Autodesk Inventor part; units mm, degrees
ref_plane "YZ Plane" through (0, 0, 0) normal (1, 0, 0) x (0, 1, 0)
ref_plane "XZ Plane" through (0, 0, 0) normal (0, 1, 0) x (-1, 0, 0)
ref_plane "XY Plane" through (0, 0, 0) normal (0, 0, 1) x (1, 0, 0)
sketch "Sketch1" plane through (0, 0, 0) normal (0, 1, 0) x (-1, 0, 0)
  arc A0 (-5.66, 120.49) -> (-5.66, 124.19) centre (-5.66, 122.34) ccw
  arc A1 (-5.66, 124.19) -> (-5.66, 120.49) centre (-5.66, 122.34) ccw
  arc A2 (5.66, 120.49) -> (5.66, 124.19) centre (5.66, 122.34) ccw
  arc A3 (5.66, 124.19) -> (5.66, 120.49) centre (5.66, 122.34) ccw
  arc A4 (0, 134.15) -> (0, 137.85) centre (0, 136) ccw
  arc A5 (0, 137.85) -> (0, 134.15) centre (0, 136) ccw
  arc A6 (-5.66, 131.81) -> (-5.66, 135.51) centre (-5.66, 133.66) ccw
  arc A7 (-5.66, 135.51) -> (-5.66, 131.81) centre (-5.66, 133.66) ccw
  arc A8 (5.66, 131.81) -> (5.66, 135.51) centre (5.66, 133.66) ccw
  arc A9 (5.66, 135.51) -> (5.66, 131.81) centre (5.66, 133.66) ccw
  arc A10 (8, 126.15) -> (8, 129.85) centre (8, 128) ccw
  arc A11 (8, 129.85) -> (8, 126.15) centre (8, 128) ccw
  arc A12 (0, 124) -> (0, 132) centre (0, 128) ccw
  arc A13 (0, 132) -> (0, 124) centre (0, 128) ccw
  arc A14 (-8, 126.15) -> (-8, 129.85) centre (-8, 128) ccw
  arc A15 (-8, 129.85) -> (-8, 126.15) centre (-8, 128) ccw
  arc A16 (0, 118.15) -> (0, 121.85) centre (0, 120) ccw
  arc A17 (0, 121.85) -> (0, 118.15) centre (0, 120) ccw
  arc A18 (-5.66, 195.81) -> (-5.66, 199.51) centre (-5.66, 197.66) ccw
  arc A19 (-5.66, 199.51) -> (-5.66, 195.81) centre (-5.66, 197.66) ccw
  arc A20 (-5.66, 184.49) -> (-5.66, 188.19) centre (-5.66, 186.34) ccw
  arc A21 (-5.66, 188.19) -> (-5.66, 184.49) centre (-5.66, 186.34) ccw
  arc A22 (5.66, 184.49) -> (5.66, 188.19) centre (5.66, 186.34) ccw
  arc A23 (5.66, 188.19) -> (5.66, 184.49) centre (5.66, 186.34) ccw
  arc A24 (5.66, 195.81) -> (5.66, 199.51) centre (5.66, 197.66) ccw
  arc A25 (5.66, 199.51) -> (5.66, 195.81) centre (5.66, 197.66) ccw
  arc A26 (8, 190.15) -> (8, 193.85) centre (8, 192) ccw
  arc A27 (8, 193.85) -> (8, 190.15) centre (8, 192) ccw
  arc A28 (-8, 190.15) -> (-8, 193.85) centre (-8, 192) ccw
  arc A29 (-8, 193.85) -> (-8, 190.15) centre (-8, 192) ccw
  arc A30 (0, 198.15) -> (0, 201.85) centre (0, 200) ccw
  arc A31 (0, 201.85) -> (0, 198.15) centre (0, 200) ccw
  arc A32 (0, 182.15) -> (0, 185.85) centre (0, 184) ccw
  arc A33 (0, 185.85) -> (0, 182.15) centre (0, 184) ccw
  arc A34 (0, 188) -> (0, 196) centre (0, 192) ccw
  arc A35 (0, 196) -> (0, 188) centre (0, 192) ccw
  arc A36 (8, 158.15) -> (8, 161.85) centre (8, 160) ccw
  arc A37 (8, 161.85) -> (8, 158.15) centre (8, 160) ccw
  arc A38 (-8, 158.15) -> (-8, 161.85) centre (-8, 160) ccw
  arc A39 (-8, 161.85) -> (-8, 158.15) centre (-8, 160) ccw
  arc A40 (0, 166.15) -> (0, 169.85) centre (0, 168) ccw
  arc A41 (0, 169.85) -> (0, 166.15) centre (0, 168) ccw
  arc A42 (0, 150.15) -> (0, 153.85) centre (0, 152) ccw
  arc A43 (0, 153.85) -> (0, 150.15) centre (0, 152) ccw
  arc A44 (0, 156) -> (0, 164) centre (0, 160) ccw
  arc A45 (0, 164) -> (0, 156) centre (0, 160) ccw
  arc A46 (-5.66, 248.49) -> (-5.66, 252.19) centre (-5.66, 250.34) ccw
  arc A47 (-5.66, 252.19) -> (-5.66, 248.49) centre (-5.66, 250.34) ccw
  arc A48 (5.66, 248.49) -> (5.66, 252.19) centre (5.66, 250.34) ccw
  arc A49 (5.66, 252.19) -> (5.66, 248.49) centre (5.66, 250.34) ccw
  arc A50 (0, 262.15) -> (0, 265.85) centre (0, 264) ccw
  arc A51 (0, 265.85) -> (0, 262.15) centre (0, 264) ccw
  arc A52 (-5.66, 259.81) -> (-5.66, 263.51) centre (-5.66, 261.66) ccw
  arc A53 (-5.66, 263.51) -> (-5.66, 259.81) centre (-5.66, 261.66) ccw
  arc A54 (5.66, 259.81) -> (5.66, 263.51) centre (5.66, 261.66) ccw
  arc A55 (5.66, 263.51) -> (5.66, 259.81) centre (5.66, 261.66) ccw
  arc A56 (8, 254.15) -> (8, 257.85) centre (8, 256) ccw
  arc A57 (8, 257.85) -> (8, 254.15) centre (8, 256) ccw
  arc A58 (0, 252) -> (0, 260) centre (0, 256) ccw
  arc A59 (0, 260) -> (0, 252) centre (0, 256) ccw
  arc A60 (8, 222.15) -> (8, 225.85) centre (8, 224) ccw
  arc A61 (8, 225.85) -> (8, 222.15) centre (8, 224) ccw
  arc A62 (-8, 222.15) -> (-8, 225.85) centre (-8, 224) ccw
  arc A63 (-8, 225.85) -> (-8, 222.15) centre (-8, 224) ccw
  arc A64 (0, 230.15) -> (0, 233.85) centre (0, 232) ccw
  arc A65 (0, 233.85) -> (0, 230.15) centre (0, 232) ccw
  arc A66 (0, 214.15) -> (0, 217.85) centre (0, 216) ccw
  arc A67 (0, 217.85) -> (0, 214.15) centre (0, 216) ccw
  arc A68 (0, 220) -> (0, 228) centre (0, 224) ccw
  arc A69 (0, 228) -> (0, 220) centre (0, 224) ccw
  arc A70 (0, 140) -> (0, 148) centre (0, 144) ccw
  arc A71 (0, 148) -> (0, 140) centre (0, 144) ccw
  arc A72 (0.1754, 172) -> (0.1754, 180) centre (0.1754, 176) ccw
  arc A73 (0.1754, 180) -> (0.1754, 172) centre (0.1754, 176) ccw
  arc A74 (0, 204) -> (0, 212) centre (0, 208) ccw
  arc A75 (0, 212) -> (0, 204) centre (0, 208) ccw
  arc A76 (0, 236) -> (0, 244) centre (0, 240) ccw
  arc A77 (0, 244) -> (0, 236) centre (0, 240) ccw
  arc A78 (-8, 254.15) -> (-8, 257.85) centre (-8, 256) ccw
  arc A79 (-8, 257.85) -> (-8, 254.15) centre (-8, 256) ccw
  arc A80 (0, 246.15) -> (0, 249.85) centre (0, 248) ccw
  arc A81 (0, 249.85) -> (0, 246.15) centre (0, 248) ccw
  arc A82 (13.5, 256) -> (0, 269.5) centre (0, 256) ccw
  arc A83 (0, 269.5) -> (-13.5, 256) centre (0, 256) ccw
  line L0 (-13.5, 256) -> (-13.5, 128)
  line L1 (13.5, 128) -> (13.5, 256)
  arc A84 (2.852, 141.1953) -> (-2.852, 141.1953) centre (0, 128) ccw
  arc A85 (-13.5, 128) -> (13.5, 128) centre (0, 128) ccw
  point P0 (0, 0)
  point P1 (0, 128)
extrude "Extrusion1" add sketch "Sketch1" along normal blind 2
sketch "Sketch2" plane through (0, 2, 0) normal (0, 1, 0) x (1, 0, 0)
  line L0 (-13.5, -128) -> (-13.5, -256)
  line L1 (-13.5, -148.6948) -> (13.5, -148.6948)
  line L2 (13.5, -148.6948) -> (13.5, -110.804)
  line L3 (13.5, -110.804) -> (-13.5, -110.804)
  line L4 (-13.5, -110.804) -> (-13.5, -148.6948)
  point P0 (0, 0)
extrude "Extrusion2" cut sketch "Sketch2" against normal blind 25.4
properties part number "Tetrix Flat bar 160 mm"
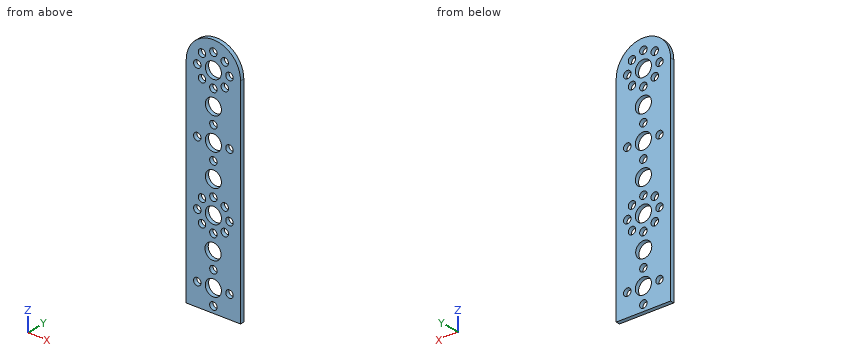
Source: CAD feature listing. Evaluate the final solid. Frame: model axes, mm. Give positions to 0.01 mm unless a question says otherwise; leave off trailing zeros. Write each loop counter-clockwise with the first axis right and the second up, starting at its lowest first coordinate (ties: lowest second). Pieces come first, ordered by that corner, then holes. Notation, with made-up numbers: (33, 69) -> (78, 69) arc R35 ccw to (78, 106) -> close; hole circle Ø9 at (-31, 45). An arc over 180 degrees is marked (long way). Return JSON: item names as keys, results as strings. Group by question number.
1. Pin query (flat end, axial travel): pin 1 Ø3.5 at (x, z) = (0, 264) entering from +Y; pin 2 Ø5 at (x, z) = (8, 224) entering from -Y. Return the tip coordinate at first contact, or that it passes through.
2. Material intervals for line 1 (X direction, y = 1.2, z = 256); line 2 (X direction, y = 0.55, z = 208); line 3 (X direction, y = 0.25, z = 176), sorted ascending. Write a range as from..to.
3. Section C-C, the plane y = 1.65. Count the separate pieces of the cut face and the enclosed holes in it, then the cut area to 3 significant figures.
4. Section B-B, the plane z = 160. Output: boundary loops of the cut face in (x, y).
5. Section A-A, the plane z = 232. Output: boundary loops of the cut face in (x, y).
6. Section D-D, the plane x = 11.25. Output: boundary loops of the cut face in (y, z).
Determined:
{
 "1": {"pin 1": "passes through", "pin 2": "stops at y = 0"},
 "2": {"line 1": "x = -13.5..-9.85, -6.15..-4, 4..6.15, 9.85..13.5", "line 2": "x = -13.5..-4, 4..13.5", "line 3": "x = -13.5..-4.18, 3.82..13.5"},
 "3": {"separate pieces": "1", "enclosed holes": "31", "area": "2,570 mm2"},
 "4": {"outline": "(-13.5, 0) -> (-9.85, 0) -> (-9.85, 2) -> (-13.5, 2) -> close; (-6.15, 0) -> (-4, 0) -> (-4, 2) -> (-6.15, 2) -> close; (4, 0) -> (6.15, 0) -> (6.15, 2) -> (4, 2) -> close; (9.85, 0) -> (13.5, 0) -> (13.5, 2) -> (9.85, 2) -> close"},
 "5": {"outline": "(-13.5, 0) -> (-1.85, 0) -> (-1.85, 2) -> (-13.5, 2) -> close; (1.85, 0) -> (13.5, 0) -> (13.5, 2) -> (1.85, 2) -> close"},
 "6": {"outline": "(0, 148.69) -> (2, 148.69) -> (2, 263.46) -> (0, 263.46) -> close"}
}
